Can you work these out from the model? Positions are in its coordinate system, mm. A direction names the side the tool comes from. Coordinates: 2 decimals unless noted, no trailing zeros. Order: outer loops, then holes, each group sorted by start corner. A loop starts at its lowest first (then second) coordinate and runs counter-clockwise, first axis right, second up. Notation, with made-up numbers: (48.5, 51) -> (53.5, 51) arc R7 ccw to (53.5, 55) -> close; hole circle Ø4 at (25.25, 51.5). An arc over 180 degrees is marked (long way). Write item = value, one per line.
```python
from build123d import *

# Parameters (mm, degrees)
F0_W        = 1.27
F0_H        = 10.16
F1_DEPTH    = 5.08
F2_T1_DEPTH = 16.0785226281
F3_R        = 1.26999
F4_R        = 0.635
F5_DEPTH    = 5.08


# Not quite as in the source:
# - a fillet or chamfer that OpenCascade refuses, or shapes differently, is made with other operations: its cross-section is extruded or revolved along the edge and cut away or added
# - a fillet or chamfer is up to 0.001 mm smaller than in the source, because OpenCascade refuses the exact size


with BuildPart() as f1:
    # F0 (on Top) → F1 (new body)
    with BuildSketch(Plane.XY):
        with Locations((0.635, 2.7667839336)):
            Rectangle(F0_W, F0_H)
    extrude(amount=F1_DEPTH)

    # F2: fillet of radius 2.54 on 2 edges, made by hand

    # F2_s2 → F2_t1 (cut)
    with BuildSketch(Plane.XY.offset(-5.499261314)):
        with BuildLine():
            ThreePointArc((0, 7.8467839336), (0.9297045256, 6.9170794079), (1.27, 5.6470794079))
            Line((1.27, 5.6470794079), (1.27, 7.8467839336))
            Line((1.27, 7.8467839336), (0, 7.8467839336))
        make_face()
        with BuildLine():
            ThreePointArc((0, -2.3132160664), (0.9297045256, -1.3835115408), (1.27, -0.1135115408))
            Line((1.27, -0.1135115408), (1.27, -2.3132160664))
            Line((1.27, -2.3132160664), (0, -2.3132160664))
        make_face()
    extrude(amount=F2_T1_DEPTH, mode=Mode.SUBTRACT)

    # F3 (radius 1.27 in the source; OpenCascade refuses exactly that, so slightly less here)
    f3_edges = [f1.edges().sort_by_distance(p)[0] for p in [
        (0.929705, 6.917079, 5.08),
        (1.27, 2.766784, 5.08),
        (0.929705, -1.383512, 5.08),
        (0.929705, 6.917079, 0),
        (0.929705, -1.383512, 0),
        (1.27, 2.766784, 0),
    ]]
    fillet(f3_edges, radius=F3_R)

    # F4 (on face) → F5 (join)
    with BuildSketch(Plane(origin=(0, 0, 0), x_dir=(0, -1, 0), z_dir=(-1, 0, 0))):
        with Locations((-2.7667839336, 2.54)):
            Circle(F4_R)
    extrude(amount=F5_DEPTH)


solid = f1.part
```
Item 1: I want a section at C-C, the plane x = -0.5. Please give me the cut outline in (y, z) (3 decimals).
A:
outline = circle Ø1.27 at (2.767, 2.54)
Item 2: For faces 1 (the cylindrical face through (-2.5, 3.27, 2.15)), 2 (the cylindrical face through (0.92, -1.4, 2.52)), which set-ups out of +Z, -Z, +X, -X, +Y, -Y let a thin tool reach every point of the face, with its end or its side?
A:
face_1 = -X
face_2 = +Z, -Z, +X, -Y
Item 3: I want a section at A-A, the plane z = 2.54. Please give me the cut outline in (x, y), plus the area to 3 significant figures.
A:
outline = (-5.08, 2.13) -> (0, 2.13) -> (0, -2.31) arc R2.54 ccw to (1.27, -0.11) -> (1.27, 5.65) arc R2.54 ccw to (0, 7.85) -> (0, 3.4) -> (-5.08, 3.4) -> close
area = 17.7 mm2
Item 4: I want a section at D-D, the plane z = 3.4. Please give me the cut outline in (x, y), plus the area to 3 significant figures.
A:
outline = (0, -2.31) arc R2.54 ccw to (1.27, -0.11) -> (1.27, 5.65) arc R2.54 ccw to (0, 7.85) -> close
area = 11.3 mm2
Item 5: If I drill on probe 1 along X at (y, z) = (3.5, 2.8); probe 2 along X at (y, z) = (1, 4.45); probe 3 along Z at (x, y) = (-4.5, 3.25), over which ranges is the centre line in solid material (lowest first)?
A:
probe_1 = 0 to 1.27
probe_2 = 0 to 1.1
probe_3 = 2.13 to 2.95
